Could you check a few things on this model? Use its own coordinates, in mm. Face numbers are marked on the shaded views. A direction names the side the tool comes from. Coordinates: 2 decimals unless noted, no trailing zeros. Order: outer loops, then holes, each group sorted by start corner. A loop starts at its lowest first (then second) coordinate and runs counter-clockwise, first axis right, second up. Notation, with made-up numbers: (58.25, 31) -> (100.25, 31) arc R11 ccw to (100.25, 40) -> close; hole circle Ø2 at (81.25, -10.75). An arc over 180 degrees is marked (long way). Use a Markdown table: item, result. Add a question column.
1) If we section it at A-A (x = 28.7): Write out the boundary of the cut face in (y, z) (3 decimals), plus the area to 3 significant figures.
2) If I drill on L1, parallel to Z at x = 9.5, y = 44; L2, parallel to Z at x = 32, y = 33.5, over which ranges is the centre line in solid material (lowest first)? Write a range as [from, to].
3) If we section it at C-C (z = 7): Write out the boundary of the cut face in (x, y) (3 decimals), plus the area to 3 significant figures.
4) If we section it at D-D (x = 44): Write out the boundary of the cut face in (y, z), plus the area to 3 significant figures.
5) Which directions (+Z, -Z, +X, -X, +Y, -Y) give clear straight access to the entire face, cutting with the end or side of a thin tool? Please do the marked faces 1 and 2.
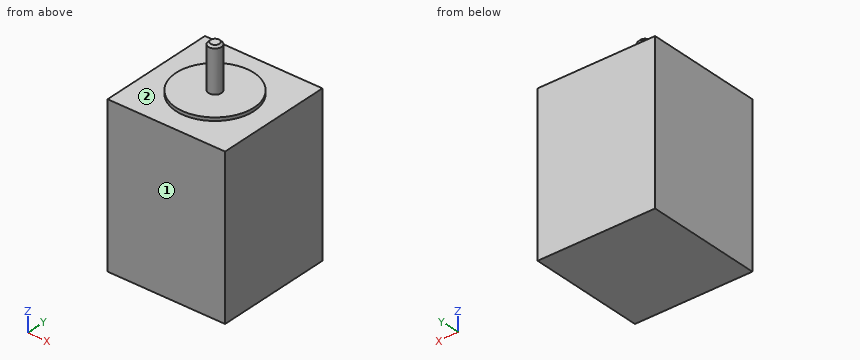
```python
from build123d import *

# Parameters (mm, degrees)
SKIZZE1_W                       = 57.4
SKIZZE1_H                       = 57.4
AUFSATZ_LINEAR_AUSTRAGEN1_DEPTH = 77
SKIZZE2_R                       = 19.065
AUFSATZ_LINEAR_AUSTRAGEN2_DEPTH = 1.6
SKIZZE3_R                       = 3.175
AUFSATZ_LINEAR_AUSTRAGEN3_DEPTH = 21.6
FASE1_SIZE                      = 1


with BuildPart() as part:
    # Skizze1 → Aufsatz-Linear austragen1 (new body)
    with BuildSketch(Plane.XY):
        with Locations((28.7, 28.7)):
            Rectangle(SKIZZE1_W, SKIZZE1_H)
    extrude(amount=-AUFSATZ_LINEAR_AUSTRAGEN1_DEPTH)

    # Skizze2 → Aufsatz-Linear austragen2 (add)
    with BuildSketch(Plane.XY):
        with Locations((28.7, 28.7)):
            Circle(SKIZZE2_R)
    extrude(amount=AUFSATZ_LINEAR_AUSTRAGEN2_DEPTH)

    # Skizze3 → Aufsatz-Linear austragen3 (add)
    with BuildSketch(Plane.XY.offset(1.6)):
        with Locations((28.7, 28.7)):
            Circle(SKIZZE3_R)
    extrude(amount=AUFSATZ_LINEAR_AUSTRAGEN3_DEPTH)

    # Fase1
    fase1_edges = [part.edges().sort_by_distance(p)[0] for p in [
        (25.525, 28.7, 23.2),
    ]]
    chamfer(fase1_edges, length=FASE1_SIZE)


solid = part.part
```
Answer sheet:
| question | item | result |
|---|---|---|
| 1 | outline | (0, -77) -> (57.4, -77) -> (57.4, 0) -> (47.765, 0) -> (47.765, 1.6) -> (31.875, 1.6) -> (31.875, 22.2) -> (30.875, 23.2) -> (26.525, 23.2) -> (25.525, 22.2) -> (25.525, 1.6) -> (9.635, 1.6) -> (9.635, 0) -> (0, 0) -> close |
| 1 | area | 4,620 mm2 |
| 2 | L1 | [-77, 0] |
| 2 | L2 | [-77, 1.6] |
| 3 | outline | circle Ø6.35 at (28.7, 28.7) |
| 3 | area | 31.7 mm2 |
| 4 | outline | (0, -77) -> (57.4, -77) -> (57.4, 0) -> (40.07, 0) -> (40.07, 1.6) -> (17.33, 1.6) -> (17.33, 0) -> (0, 0) -> close |
| 4 | area | 4,460 mm2 |
| 5 | face 1 | +Z, -Z, +X, -X, -Y |
| 5 | face 2 | +Z |
